```python
from build123d import *
from OCP.BRepFilletAPI import BRepFilletAPI_MakeFillet

# Parameters (mm, degrees)
SKETCH_1_W           = 41.5
SKETCH_1_H           = 18
EXTRUDE_1_DEPTH      = 41.5
CUT_EXTRUDE_2_DEPTH  = 41.5
CUT_EXTRUDE_3_DEPTH  = 1.5
SKETCH_4_W           = 10
SKETCH_4_H           = 42.806652411
CUT_EXTRUDE_4_DEPTH  = 1.5
SKETCH_5_W           = 46.146220502
SKETCH_5_H           = 19
SKETCH_5_W_2         = 42.146220502
SKETCH_5_H_2         = 16
CUT_EXTRUDE_5_DEPTH  = 1.5
SKETCH_6_W           = 43.828309831
SKETCH_6_H           = 10
CUT_EXTRUDE_7_DEPTH  = 1.5
FILLET_8_R1          = 5
FILLET_8_R2          = 6.5
CHAMFER_1_SIZE       = 1.5
CUT_EXTRUDE_9_DEPTH  = 13
SKETCH_10_R          = 3.5
CUT_EXTRUDE_10_DEPTH = 10
SKETCH_11_R          = 3.5
CUT_EXTRUDE_11_DEPTH = 5
SKETCH_12_R          = 1.75
CUT_EXTRUDE_12_DEPTH = 20


with BuildPart() as part:
    # 草图1 → 拉伸1 (new body)
    with BuildSketch(Plane(origin=(0, 0, 0), x_dir=(1, 0, 0), z_dir=(0, 1, 0))):
        with Locations((20.75, 9)):
            Rectangle(SKETCH_1_W, SKETCH_1_H)
    extrude(amount=EXTRUDE_1_DEPTH)

    # 草图2 → 拉伸2 (cut)
    with BuildSketch(Plane.XY):
        Polygon((5, 41.5), (41.5, 41.5), (41.5, 5), (35, 5), (5, 35), align=None)
    extrude(amount=-CUT_EXTRUDE_2_DEPTH, mode=Mode.SUBTRACT)

    # 草图3 → 拉伸3 (cut)
    with BuildSketch(Plane.ZY):
        Polygon((1.5, 43), (1.5, -2.474095728), (-1, -2.474095728), (-1, 40), (-17, 40), (-17, -2.474095728), (-19.5, -2.474095728), (-19.5, 43), align=None)
    extrude(amount=-CUT_EXTRUDE_3_DEPTH, mode=Mode.SUBTRACT)

    # 草图4 → 拉伸4 (cut)
    with BuildSketch(Plane.ZY):
        with Locations((-9, 20.096673794)):
            Rectangle(SKETCH_4_W, SKETCH_4_H)
    extrude(amount=-CUT_EXTRUDE_4_DEPTH, mode=Mode.SUBTRACT)

    # 草图5 → 拉伸5 (cut)
    with BuildSketch(Plane.XZ):
        with Locations((19.426889749, -9)):
            Rectangle(SKETCH_5_W, SKETCH_5_H)
        with Locations((18.926889749, -9)):
            Rectangle(SKETCH_5_W_2, SKETCH_5_H_2, mode=Mode.SUBTRACT)
    extrude(amount=-CUT_EXTRUDE_5_DEPTH, mode=Mode.SUBTRACT)

    # 草图6 → 拉伸7 (cut)
    with BuildSketch(Plane.XZ):
        with Locations((19.585845085, -9)):
            Rectangle(SKETCH_6_W, SKETCH_6_H)
    extrude(amount=-CUT_EXTRUDE_7_DEPTH, mode=Mode.SUBTRACT)

    # 圆角8: one fillet with a radius per group of edges: ONE call of the kernel's fillet builder (fillet() takes one radius for all edges)
    fillet_8_edges_1 = [part.edges().sort_by_distance(p)[0] for p in [
        (1.5, 1.5, -17.5),
        (1.5, 1.5, -9),
        (1.5, 1.5, -0.5),
    ]]
    fillet_8_edges_2 = [part.edges().sort_by_distance(p)[0] for p in [
        (0, 0, -15.5),
        (0, 0, -2.5),
    ]]
    fillet_8 = BRepFilletAPI_MakeFillet(part.part.solid().wrapped)
    for e in fillet_8_edges_1:
        fillet_8.Add(FILLET_8_R1, e.wrapped)
    for e in fillet_8_edges_2:
        fillet_8.Add(FILLET_8_R2, e.wrapped)
    add(Compound.cast(fillet_8.Shape()), mode=Mode.REPLACE)

    # 倒角1
    chamfer_1_edges = [part.edges().sort_by_distance(p)[0] for p in [
        (0, 40, -2.5),
        (0, 40, -15.5),
        (40, 0, -2.5),
        (40, 0, -15.5),
    ]]
    chamfer(chamfer_1_edges, length=CHAMFER_1_SIZE - 0.0001)  # a hair under: the kernel refuses the full size

    # 草图9 → 拉伸9 (cut)
    with BuildSketch(Plane(origin=(0, 0, -15.5), x_dir=(-1, 0, 0), z_dir=(0, 0, -1))):
        Polygon((-5, 38.898928625), (-5, 9.5), (-9.5, 5), (-37.05605145, 5), (-37.05605145, 38.898928625), align=None)
    extrude(amount=-CUT_EXTRUDE_9_DEPTH, mode=Mode.SUBTRACT)

    # 草图10 → 拉伸10 (cut)
    with BuildSketch(Plane.XZ.offset(-1.5)):
        with Locations(Location((21.5, -9, 0), (0, 0, 270))):
            Circle(SKETCH_10_R)
        with Locations(Location((36.5, -9, 0), (0, 0, 270))):
            Circle(SKETCH_10_R)
    extrude(amount=-CUT_EXTRUDE_10_DEPTH, mode=Mode.SUBTRACT)

    # 草图11 → 拉伸11 (cut)
    with BuildSketch(Plane.ZY.offset(-1.5)):
        with Locations((-9, 21.5)):
            Circle(SKETCH_11_R)
        with Locations((-9, 36.5)):
            Circle(SKETCH_11_R)
    extrude(amount=-CUT_EXTRUDE_11_DEPTH, mode=Mode.SUBTRACT)

    # 草图12 → 拉伸12 (cut)
    with BuildSketch(Plane.XY):
        with Locations((11.75, 11.75)):
            Circle(SKETCH_12_R)
    extrude(amount=-CUT_EXTRUDE_12_DEPTH, mode=Mode.SUBTRACT)


solid = part.part
```
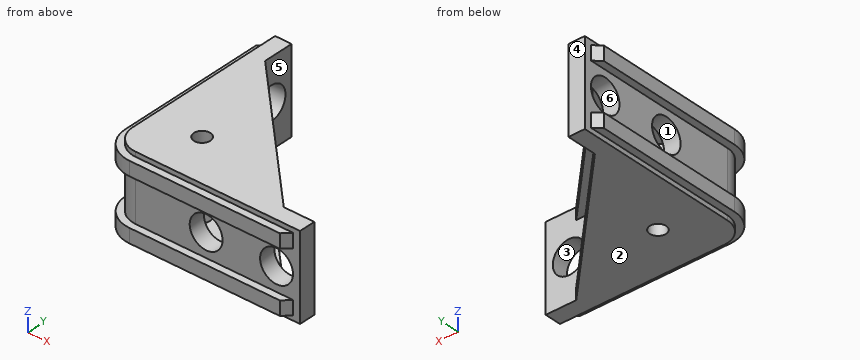
Model file for the job. Use its own axes, mm. Face numbers are marked on the shaded views. A direction names the side the tool comes from. Give positions to 0.01 mm unless a question says otherwise; leave off trailing zeros. Write each loop counter-clockwise with the first axis right and the second up, starting at its lowest first coordinate (ties: lowest second). Pieces come first, ordered by that corner, then holes. Notation, with made-up numbers: (67, 30.25) - (100, 30.25) arc R19 ccw to (100, 46.25) - close; hole circle Ø1 at (0.25, -36.75). An arc over 180 degrees is marked (long way). One line per question, with ' | ' between items. Start each with the question number.
(1) 3-axis set-ups, long thin cutter, end or side, ignore diameter. For the marked faces 5 and 6: which of +Z, -Z, +X, -X, +Y, -Y reach the whole face in a straight line?
(2) Pin check, flat tips, straight feed: P1, Ø8, axis at x = 25, z = -15.5, coming from the +Y side; P2, Ø2, axis at x = 11.75, y = 11.75, coming from the -Z side; P3, Ø1.5, axis at x = 9.5, z = -14, coming from the +Y side; P4, Ø8, axis at y = 21.5, z = -9, coming from the -X side. Stop position of each tip, or through.
(3) Wall check: line 1 along Z through (x, y) = (23.5, 13.5); line 2 along X through (y, z) = (3.7, -9); line 3 along X through (y, z) = (3.5, -10.75). Give the ranges that are in metal, low to high. Write a range as from..to.
(4) Slice it at A-A on x = 36.5. Write the cut outline in (y, z), plus the area to 3 significant figures.
(5) Slice it at B-B on y = 11.75. Write the cut outline in (x, z), plus the area to 3 significant figures.
(6) Slice it at C-C on z = -9. Write the cut outline in (x, y).
(7) Two-plate mould, pull along Z, no slides. Class the marked faces 1, 2, 3 and 4: +Z half, -Z half, draft (parallel to the pull), parting line (faces both ways), or undercut.
Results below:
1) face 5: +X, +Y | face 6: +X, -X
2) P1: y = 19 | P2: through | P3: y = 5.75 | P4: x = 1.5
3) line 1: -18..-15.5, -2.5..0 | line 2: 2.36..18, 25..33, 40..41.5 | line 3: 2.5..18.47, 24.53..33.47, 39.53..41.5
4) outline: (0, -17) - (1.5, -17) - (1.5, -18) - (5, -18) - (5, -12.5) - (1.5, -12.5) - (1.5, -14) - (0, -14) - close; (0, -4) - (1.5, -4) - (1.5, -5.5) - (5, -5.5) - (5, 0) - (1.5, 0) - (1.5, -1) - (0, -1) - close | area: 47.5 mm^2
5) outline: (0, -17) - (1.5, -17) - (1.5, -18) - (10, -18) - (10, -15.5) - (5, -15.5) - (5, -2.5) - (10, -2.5) - (10, 0) - (1.5, 0) - (1.5, -1) - (0, -1) - (0, -4) - (1.5, -4) - (1.5, -14) - (0, -14) - close; (13.5, -18) - (28.25, -18) - (28.25, -15.5) - (13.5, -15.5) - close; (13.5, -2.5) - (28.25, -2.5) - (28.25, 0) - (13.5, 0) - close | area: 171 mm^2
6) outline: (1.5, 6.5) arc R5 ccw to (6.5, 1.5) - (18, 1.5) - (18, 5) - (9.5, 5) - (5, 9.5) - (5, 18) - (1.5, 18) - close; (1.5, 25) - (5, 25) - (5, 33) - (1.5, 33) - close; (1.5, 40) - (5, 40) - (5, 41.5) - (1.5, 41.5) - close; (25, 1.5) - (33, 1.5) - (33, 5) - (25, 5) - close; (40, 1.5) - (41.5, 1.5) - (41.5, 5) - (40, 5) - close
7) face 1: undercut | face 2: -Z half | face 3: undercut | face 4: draft
